from build123d import *

# Parameters (mm, degrees)
SKETCH_1_W           = 40
SKETCH_1_H           = 29
EXTRUDE_1_DEPTH      = 3
CUT_EXTRUDE_1_DEPTH  = 3
SKETCH_3_W           = 40
SKETCH_3_H           = 3
EXTRUDE_2_DEPTH      = 10
SKETCH_4_W           = 40
SKETCH_4_H           = 3
EXTRUDE_3_DEPTH      = 10
SKETCH_6_W           = 3
SKETCH_6_H           = 49
EXTRUDE_5_DEPTH      = 42
SKETCH_8_W           = 3
SKETCH_8_H           = 49
EXTRUDE_6_DEPTH      = 2
SKETCH_9_W           = 3
SKETCH_9_H           = 49
EXTRUDE_7_DEPTH      = 2
SKETCH_10_W          = 86
SKETCH_10_H          = 3
EXTRUDE_8_DEPTH      = 10
SKETCH_11_W          = 86
SKETCH_11_H          = 3
EXTRUDE_9_DEPTH      = 10
SKETCH_14_W          = 3
SKETCH_14_H          = 69
CUT_EXTRUDE_5_DEPTH  = 43
SKETCH_17_W          = 43
SKETCH_17_H          = 3
EXTRUDE_10_DEPTH     = 20
SKETCH_18_R          = 2.1
CUT_EXTRUDE_6_DEPTH  = 10
SKETCH_20_W          = 43
SKETCH_20_H          = 3
EXTRUDE_11_DEPTH     = 10
SKETCH_21_W          = 43
SKETCH_21_H          = 3
CUT_EXTRUDE_7_DEPTH  = 20
SKETCH_24_R          = 2.2
CUT_EXTRUDE_8_DEPTH  = 30
SKETCH_27_R          = 1.6
CUT_EXTRUDE_9_DEPTH  = 10
SKETCH_28_W          = 3
SKETCH_28_H          = 79
CUT_EXTRUDE_10_DEPTH = 8
SKETCH_29_W          = 35
SKETCH_29_H          = 3
CUT_EXTRUDE_11_DEPTH = 15
M3X0_5_2_D           = 2.5
M3X0_5_2_DEPTH       = 8.5
M3X0_5_2_TIP         = 0.751075774


with BuildPart() as part:
    # ｽｹｯﾁ1 → ﾎﾞｽ - 押し出し1 (new body)
    with BuildSketch(Plane.XY):
        Rectangle(SKETCH_1_W, SKETCH_1_H)
    extrude(amount=EXTRUDE_1_DEPTH)

    # ｽｹｯﾁ2 → ｶｯﾄ - 押し出し1 (cut)
    with BuildSketch(Plane.XY.offset(3)):
        with BuildLine():
            ThreePointArc((-14.4, 10.5), (-15.01507576, 11.98492424), (-16.5, 12.6))
            Line((-16.5, 12.6), (-16.5, 10.5))
            Line((-16.5, 10.5), (-18.6, 10.5))
            ThreePointArc((-18.6, 10.5), (-16.5, 8.4), (-14.4, 10.5))
        make_face()
        with BuildLine():
            Line((-16.5, 10.5), (-16.5, 12.6))
            ThreePointArc((-16.5, 12.6), (-17.98492424, 11.98492424), (-18.6, 10.5))
            Line((-18.6, 10.5), (-16.5, 10.5))
        make_face()
        with BuildLine():
            ThreePointArc((-18.6, -10.5), (-17.98492424, -11.98492424), (-16.5, -12.6))
            Line((-16.5, -12.6), (-16.5, -10.5))
            Line((-16.5, -10.5), (-18.6, -10.5))
        make_face()
        with BuildLine():
            Line((-16.5, -10.5), (-16.5, -12.6))
            ThreePointArc((-16.5, -12.6), (-15.01507576, -11.98492424), (-14.4, -10.5))
            ThreePointArc((-14.4, -10.5), (-16.5, -8.4), (-18.6, -10.5))
            Line((-18.6, -10.5), (-16.5, -10.5))
        make_face()
        with BuildLine():
            ThreePointArc((18.6, -10.5), (15.01507576, -9.01507576), (16.5, -12.6))
            Line((16.5, -12.6), (16.5, -10.5))
            Line((16.5, -10.5), (18.6, -10.5))
        make_face()
        with BuildLine():
            Line((16.5, -10.5), (16.5, -12.6))
            ThreePointArc((16.5, -12.6), (17.98492424, -11.98492424), (18.6, -10.5))
            Line((18.6, -10.5), (16.5, -10.5))
        make_face()
        with BuildLine():
            ThreePointArc((18.6, 10.5), (17.98492424, 11.98492424), (16.5, 12.6))
            Line((16.5, 12.6), (16.5, 10.5))
            Line((16.5, 10.5), (18.6, 10.5))
        make_face()
        with BuildLine():
            Line((16.5, 10.5), (16.5, 12.6))
            ThreePointArc((16.5, 12.6), (15.01507576, 9.01507576), (18.6, 10.5))
            Line((18.6, 10.5), (16.5, 10.5))
        make_face()
    extrude(amount=-CUT_EXTRUDE_1_DEPTH, mode=Mode.SUBTRACT)

    # ｽｹｯﾁ3 → ﾎﾞｽ - 押し出し2 (add)
    with BuildSketch(Plane.XZ.offset(14.5)):
        with Locations((0, 1.5)):
            Rectangle(SKETCH_3_W, SKETCH_3_H)
    extrude(amount=EXTRUDE_2_DEPTH)

    # ｽｹｯﾁ4 → ﾎﾞｽ - 押し出し3 (add)
    with BuildSketch(Plane(origin=(0, 14.5, 0), x_dir=(1, 0, 0), z_dir=(0, 1, 0))):
        with Locations((0, -1.5)):
            Rectangle(SKETCH_4_W, SKETCH_4_H)
    extrude(amount=EXTRUDE_3_DEPTH)

    # ｽｹｯﾁ6 → ﾎﾞｽ - 押し出し5 (add)
    with BuildSketch(Plane(origin=(20, 0, 0), x_dir=(0, 0, -1), z_dir=(1, 0, 0))):
        with Locations((-1.5, 0)):
            Rectangle(SKETCH_6_W, SKETCH_6_H)
    extrude(amount=EXTRUDE_5_DEPTH)

    # ｽｹｯﾁ8 → ﾎﾞｽ - 押し出し6 (add)
    with BuildSketch(Plane.ZY.offset(20)):
        with Locations((1.5, 0)):
            Rectangle(SKETCH_8_W, SKETCH_8_H)
    extrude(amount=EXTRUDE_6_DEPTH)

    # ｽｹｯﾁ9 → ﾎﾞｽ - 押し出し7 (add)
    with BuildSketch(Plane(origin=(62, 0, 0), x_dir=(0, 0, -1), z_dir=(1, 0, 0))):
        with Locations((-1.5, 0)):
            Rectangle(SKETCH_9_W, SKETCH_9_H)
    extrude(amount=EXTRUDE_7_DEPTH)

    # ｽｹｯﾁ10 → ﾎﾞｽ - 押し出し8 (add)
    with BuildSketch(Plane.XZ.offset(24.5)):
        with Locations((21, 1.5)):
            Rectangle(SKETCH_10_W, SKETCH_10_H)
    extrude(amount=EXTRUDE_8_DEPTH)

    # ｽｹｯﾁ11 → ﾎﾞｽ - 押し出し9 (add)
    with BuildSketch(Plane(origin=(0, 24.5, 0), x_dir=(1, 0, 0), z_dir=(0, 1, 0))):
        with Locations((21, -1.5)):
            Rectangle(SKETCH_11_W, SKETCH_11_H)
    extrude(amount=EXTRUDE_9_DEPTH)

    # ｽｹｯﾁ14 → ｶｯﾄ - 押し出し5 (cut)
    with BuildSketch(Plane.ZY.offset(22)):
        with Locations((1.5, 0)):
            Rectangle(SKETCH_14_W, SKETCH_14_H)
    extrude(amount=-CUT_EXTRUDE_5_DEPTH, mode=Mode.SUBTRACT)

    # ｽｹｯﾁ17 → ﾎﾞｽ - 押し出し10 (add)
    with BuildSketch(Plane.XZ.offset(34.5)):
        with Locations((42.5, 1.5)):
            Rectangle(SKETCH_17_W, SKETCH_17_H)
    extrude(amount=EXTRUDE_10_DEPTH)

    # ｽｹｯﾁ18 → ｶｯﾄ - 押し出し6 (cut)
    with BuildSketch(Plane.XY.offset(3)):
        with Locations((36, -34.5)):
            Circle(SKETCH_18_R)
        with Locations((57, -34.5)):
            Circle(SKETCH_18_R)
    extrude(amount=-CUT_EXTRUDE_6_DEPTH, mode=Mode.SUBTRACT)

    # ｽｹｯﾁ20 → ﾎﾞｽ - 押し出し11 (add)
    with BuildSketch(Plane.XZ.offset(54.5)):
        with Locations((42.5, 1.5)):
            Rectangle(SKETCH_20_W, SKETCH_20_H)
    extrude(amount=EXTRUDE_11_DEPTH)

    # ｽｹｯﾁ21 → ｶｯﾄ - 押し出し7 (cut)
    with BuildSketch(Plane.XZ.offset(64.5)):
        with Locations((42.5, 1.5)):
            Rectangle(SKETCH_21_W, SKETCH_21_H)
    extrude(amount=-CUT_EXTRUDE_7_DEPTH, mode=Mode.SUBTRACT)

    # ｽｹｯﾁ24 → ｶｯﾄ - 押し出し8 (cut)
    with BuildSketch(Plane(origin=(0, 0, 0), x_dir=(-1, 0, 0), z_dir=(0, 0, -1))):
        with Locations((-36.27, 14.5)):
            Circle(SKETCH_24_R)
        with Locations((-57, 14.5)):
            Circle(SKETCH_24_R)
    extrude(amount=-CUT_EXTRUDE_8_DEPTH, mode=Mode.SUBTRACT)

    # ｽｹｯﾁ27 → ｶｯﾄ - 押し出し9 (cut)
    with BuildSketch(Plane(origin=(0, 0, 0), x_dir=(-1, 0, 0), z_dir=(0, 0, -1))):
        with Locations((-36.11, -7.5)):
            Circle(SKETCH_27_R)
    extrude(amount=-CUT_EXTRUDE_9_DEPTH, mode=Mode.SUBTRACT)

    # ｽｹｯﾁ28 → ｶｯﾄ - 押し出し10 (cut)
    with BuildSketch(Plane.ZY.offset(-21)):
        with Locations((1.5, -5)):
            Rectangle(SKETCH_28_W, SKETCH_28_H)
    extrude(amount=-CUT_EXTRUDE_10_DEPTH, mode=Mode.SUBTRACT)

    # ｽｹｯﾁ29 → ｶｯﾄ - 押し出し11 (cut)
    with BuildSketch(Plane(origin=(0, 34.5, 0), x_dir=(1, 0, 0), z_dir=(0, 1, 0))):
        with Locations((46.5, -1.5)):
            Rectangle(SKETCH_29_W, SKETCH_29_H)
    extrude(amount=-CUT_EXTRUDE_11_DEPTH, mode=Mode.SUBTRACT)

    # M3x0.5 ねじ穴2
    with Locations(Plane(origin=(31.47, -21.64, 3), x_dir=(1, 0, 0), z_dir=(0, 0, 1))):
        with Locations((0, 0), (22.2, 10.3)):
            Hole(M3X0_5_2_D / 2, depth=M3X0_5_2_DEPTH)
            with Locations((0, 0, -(M3X0_5_2_DEPTH + M3X0_5_2_TIP / 2))):  # 118° drill point
                Cone(0, M3X0_5_2_D / 2, M3X0_5_2_TIP, mode=Mode.SUBTRACT)


solid = part.part
Can you work these out from the model? Positions are in its coordinate system, mm. Give positions to 0.01 mm unless a question says otherwise; leave off trailing zeros. Write each loop counter-clockwise with the first axis right and the second up, starting at its lowest first coordinate (ties: lowest second). Pieces come first, ordered by that corner, then holes. Notation, with made-up numbers: M -36.5,79 L -21.5,79 A19 ccw -21.5,84 Z; hole C -36.5,81 d8. An arc over 180 degrees is marked long. Answer in a Markdown table with one row per item. Add a question column.
Item 1: Imagine slicing it at C-C, the plane z = 2.1. Write out the boundary of the cut face in (x, y).
Item 2: Please list where these lines run through material, in increasing order: L1, parallel to Y at x = 57, z = 1.1; L2, parallel to Y at x = 36.27, z = 0.8; L3, parallel to Y at x = 31.47, z = 1.5.
Item 3: Imagine slicing it at A-A, the plane x = 53.67. Write out the boundary of the cut face in (y, z), plus the area to 4 significant figures.
Item 4: Imagine slicing it at B-B, the plane y = -7.5. Write out the boundary of the cut face in (x, z).
Item 5: We'd pull the mould along Y, two halves only. Please class faces 1 (the flat face through (46, -12, 3)), 2 (the flat face through (46, 19.5, 1)), 3 (the cylindrical face through (38.468, 14.597, 1.479)): released by +Y, released by -Y, zero draft, split by the parting line, or undercut.
Item 6: Imagine slicing it at D-D, the plane x = 36.5. Write out the boundary of the cut face in (y, z).
Evaluation:
| question | item | result |
|---|---|---|
| 1 | outline | M 29,-44.5 L 64,-44.5 L 64,19.5 L 29,19.5 Z; hole C 31.47,-21.64 d2.5; hole C 36,-34.5 d4.2; hole C 36.27,14.5 d4.4; hole C 36.11,-7.5 d3.2; hole C 53.67,-11.34 d2.5; hole C 57,14.5 d4.4; hole C 57,-34.5 d4.2 |
| 2 | L1 | y = -44.5 to -36.6, -32.4 to 12.3, 16.7 to 19.5 |
| 2 | L2 | y = -44.5 to -36.58, -32.42 to -9.09, -5.91 to 12.3, 16.7 to 19.5 |
| 2 | L3 | y = -44.5 to -22.89, -20.39 to 19.5 |
| 3 | outline | M -44.5,0 L -12.59,0 L -12.59,3 L -44.5,3 Z; M -10.09,0 L 19.5,0 L 19.5,3 L -10.09,3 Z |
| 3 | area | 184.5 mm² |
| 4 | outline | M 29,0 L 34.51,0 L 34.51,3 L 29,3 Z; M 37.71,0 L 64,0 L 64,3 L 37.71,3 Z |
| 5 | face 1 | zero draft |
| 5 | face 2 | released by +Y |
| 5 | face 3 | undercut |
| 6 | outline | M -44.5,0 L -36.54,0 L -36.54,3 L -44.5,3 Z; M -32.46,0 L -9.05,0 L -9.05,3 L -32.46,3 Z; M -5.95,0 L 12.31,0 L 12.31,3 L -5.95,3 Z; M 16.69,0 L 19.5,0 L 19.5,3 L 16.69,3 Z |
